Verification items for the finished model (mm, model axes). Face numbers are marked on the shaded views. Coordinates: 2 decimals unless noted, no trailing zeros. Order: outer loops, then holes, each group sorted by start corner. A loop starts at its lowest first (then second) coordinate and runs counter-clockwise, first axis right, second up. Notation, with made-up numbers: (-21, 75) -> (-7, 75) arc R37 ccw to (-7, 113) -> close; hole circle Ø5 at (-20, -16.75). An arc over 180 degrees is marked (long way). Answer as CSV lines item,"result".
```python
from build123d import *

# Parameters (mm, degrees)
F0_W     = 304.8
F0_H     = 63.5
F1_DEPTH = 39.6875
F2_SIZE2 = 304.79999
F2_SIZE  = 47.62499
F3_R     = 11.1125
F4_DEPTH = 50.8


# Not quite as in the source:
# - a fillet or chamfer is up to 0.001 mm smaller than in the source, because OpenCascade refuses the exact size
# - a length typed as a fraction of an inch, garbled in the dataset ("3 / 203.2 mm" for 3/8 in), is restored


with BuildPart() as f1:
    # F0 (on Front) → F1 (new body)
    with BuildSketch(Plane.XZ):
        with Locations((152.4, 31.75)):
            Rectangle(F0_W, F0_H)
    extrude(amount=F1_DEPTH)

    # F2 (size 47.625 and 304.8 in the source; OpenCascade refuses exactly that, so slightly less here)
    f2_edges = [f1.edges().sort_by_distance(p)[0] for p in [
        (0, -19.84375, 63.5),
    ]]
    f2_side = f1.faces().sort_by_distance((0, -19.84375, 31.75))[0]
    chamfer(f2_edges, length=F2_SIZE, length2=F2_SIZE2, reference=f2_side)

    # F3 (on face) → F4 (cut)
    with BuildSketch(Plane.YZ.offset(304.8)):
        with Locations((-19.84375, 19.05)):
            Circle(F3_R)
    extrude(amount=-F4_DEPTH, mode=Mode.SUBTRACT)


solid = f1.part
```
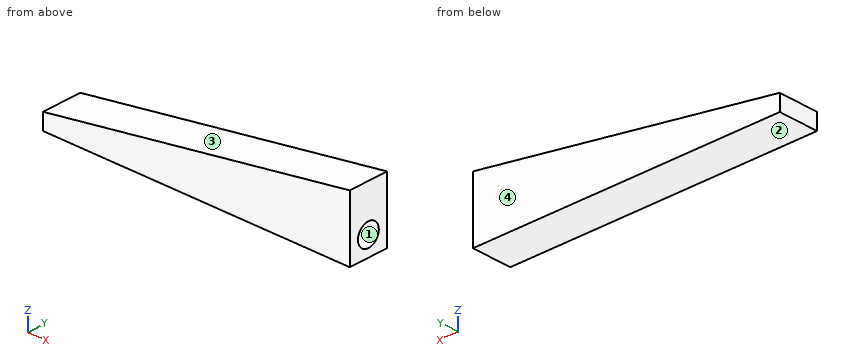
Item 1: Section check C-C, the plane z = 19.05. Record the boundary of the cut face in (x, y).
Answer list:
outline,"(20.32, -39.69) -> (304.8, -39.69) -> (304.8, -30.96) -> (254, -30.96) -> (254, -8.73) -> (304.8, -8.73) -> (304.8, 0) -> (20.32, 0) -> close"
Item 2: Depth check by flat-ended pin: pin 1 Ø20 at (y, z) = (-19.84, 19.05) entering from -X; pin 2 Ø2 at (y, z) = (-23.5, 17) entering from +X; pin 3 Ø5 at (x, y) = (38, -27.5) entering from +Z; pin 4 Ø12 at (x, y) = (171, -25) entering from +Z. Enter the tip coordinate at first touch or a pass-through.
Answer list:
pin 1,"x = 0"
pin 2,"x = 254"
pin 3,"z = 22.2"
pin 4,"z = 43.53"
Item 3: Thickness scan on line 1 (Y direction, x = 291, z = 19); line 2 (Z direction, x = 263, y = -18.5); line 3 (Z direction, x = 75.5, y = -33). Record the ranges inside material, lowest first.
Answer list:
line 1,"-39.69 to -30.96, -8.73 to 0"
line 2,"0 to 8.02, 30.08 to 56.97"
line 3,"0 to 27.67"
Item 4: Release check for a two-part mould opening along Z. For the marked faces 1, 2, 3 and 4 record: +Z half, -Z half, draft (parallel to the pull), parting line (faces both ways), or undercut.
Answer list:
face 1,"undercut"
face 2,"-Z half"
face 3,"+Z half"
face 4,"draft"
Item 5: Section check B-B, the plane x = 52. Record the boundary of the cut face in (y, z), plus the area to 4 significant figures.
Answer list:
outline,"(-39.69, 0) -> (0, 0) -> (0, 24) -> (-39.69, 24) -> close"
area,"952.5 mm2"
Item 6: Section check D-D, the plane x = 20. Record the boundary of the cut face in (y, z).
Answer list:
outline,"(-39.69, 0) -> (0, 0) -> (0, 19) -> (-39.69, 19) -> close"
